For this review, take the finished solid that the model builds, in its own axes (mm). Face numbers are marked on the shaded views. A direction names the side the tool comes from. Round coordinates to 2 decimals unless told otherwise and drop trailing zeros. Write each loop counter-clockwise with the first axis right and the second up, starting at its lowest first coordinate (ties: lowest second). Pieces come first, ordered by that corner, then holes. Notation, with made-up numbers: (61, -24) -> (119, -24) arc R28 ccw to (119, 12) -> close; hole circle Ø10 at (10, 65.25). An arc over 180 degrees is marked (long way). Write item = value, one per line. Start each with the question number.
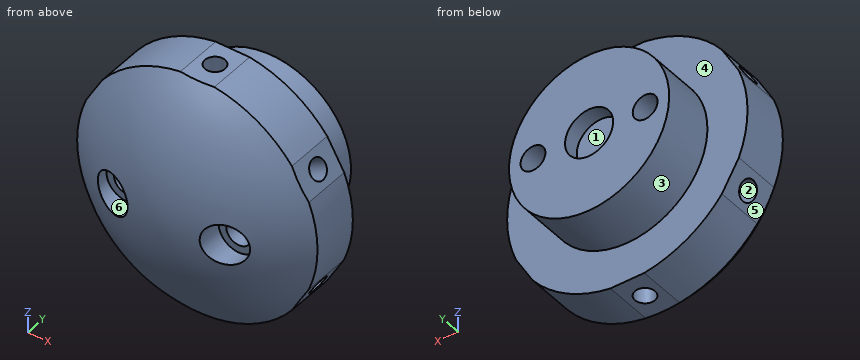
```python
from build123d import *

# Parameters (mm, degrees)
SKETCH_1_R               = 15
EXTRUDE_1_DEPTH          = 6
SKETCH_2_R               = 10
EXTRUDE_2_DEPTH          = 6.5
SKETCH_5_R               = 1.55
CUT_EXTRUDE_967_DEPTH    = 29.287523448
SKETCH_6_R               = 2.5
CUT_EXTRUDE_1129_DEPTH   = 3.7
CUT_EXTRUDE_3_DEPTH      = 25.477792773
PATTERN_CIRCULAR_1_COUNT = 6
SKETCH_12_R              = 3
CUT_EXTRUDE_4_DEPTH      = 2


with BuildPart() as part:
    # 草图1 → 凸台-拉伸1 (new body)
    with BuildSketch(Plane(origin=(0, 0, 0), x_dir=(1, 0, 0), z_dir=(0, 1, 0))):
        with Locations(Location((0, 0, 0), (0, 0, 270))):
            Circle(SKETCH_1_R)
    extrude(amount=EXTRUDE_1_DEPTH)

    # 草图2 → 凸台-拉伸2 (add)
    with BuildSketch(Plane(origin=(0, 6, 0), x_dir=(1, 0, 0), z_dir=(0, 1, 0))):
        with Locations(Location((0, 0, 0), (0, 0, 90))):
            Circle(SKETCH_2_R)
    extrude(amount=EXTRUDE_2_DEPTH)

    # 草图4 → 旋转1 (revolve)
    with BuildSketch(Plane.XY, mode=Mode.PRIVATE) as revolve_1_sk:
        with BuildLine():
            Line((0, 0), (0, -6.213203436))
            ThreePointArc((0, -6.213203436), (8.117941502, -4.598444473), (15, 0))
            Line((15, 0), (0, 0))
        make_face()
    revolve(revolve_1_sk.sketch.rotate(Axis((0, 0, 0), (0, -1, 0)), 180), axis=Axis((0, 0, 0), (0, -1, 0)))

    # 草图5 → Cut-Extrude 967 (cut, through all)
    with BuildSketch(Plane(origin=(0, 12.5, 0), x_dir=(1, 0, 0), z_dir=(0, 1, 0))):
        with Locations(Location((7, 0, 0), (0, 0, 270))):
            Circle(SKETCH_5_R)
        with Locations(Location((-7, 0, 0), (0, 0, 270))):
            Circle(SKETCH_5_R)
    extrude(amount=-CUT_EXTRUDE_967_DEPTH, mode=Mode.SUBTRACT)

    # 草图6 → Cut-Extrude 1129 (cut)
    with BuildSketch(Plane(origin=(0, -6.2, 0), x_dir=(1, 0, 0), z_dir=(0, 1, 0))):
        with Locations(Location((-7, 0, 0), (0, 0, 129.482318069))):
            Circle(SKETCH_6_R)
        with Locations(Location((7, 0, 0), (0, 0, 133.910612472))):
            Circle(SKETCH_6_R)
    extrude(amount=CUT_EXTRUDE_1129_DEPTH, mode=Mode.SUBTRACT)

    # 草图9 → 切除-拉伸3 (cut, through all)
    with BuildSketch(Plane(origin=(0, 6, 0), x_dir=(1, 0, 0), z_dir=(0, 1, 0))):
        with BuildLine():
            Line((11.802472048, 9.257518758), (13.918482445, 5.592481242))
            ThreePointArc((13.918482445, 5.592481242), (12.990381057, 7.5), (11.802472048, 9.257518758))
        make_face()
        with BuildLine():
            Line((-2.116010397, 14.85), (2.116010397, 14.85))
            ThreePointArc((2.116010397, 14.85), (0, 15), (-2.116010397, 14.85))
        make_face()
        with BuildLine():
            Line((13.918482445, -5.592481242), (11.802472048, -9.257518758))
            ThreePointArc((11.802472048, -9.257518758), (12.990381057, -7.5), (13.918482445, -5.592481242))
        make_face()
        with BuildLine():
            Line((2.116010397, -14.85), (-2.116010397, -14.85))
            ThreePointArc((-2.116010397, -14.85), (0, -15), (2.116010397, -14.85))
        make_face()
        with BuildLine():
            Line((-11.802472048, -9.257518758), (-13.918482445, -5.592481242))
            ThreePointArc((-13.918482445, -5.592481242), (-12.990381057, -7.5), (-11.802472048, -9.257518758))
        make_face()
        with BuildLine():
            Line((-13.918482445, 5.592481242), (-11.802472048, 9.257518758))
            ThreePointArc((-11.802472048, 9.257518758), (-12.990381057, 7.5), (-13.918482445, 5.592481242))
        make_face()
    extrude(amount=-CUT_EXTRUDE_3_DEPTH, mode=Mode.SUBTRACT)

    # 草图11 → M3 螺纹孔2 (revolve, cut)
    with BuildSketch(Plane(origin=(-12.860477246, 3, -7.425), x_dir=(-0.50000000000004, 0, 0.8660254037844157), z_dir=(0, 1, 0))):
        Polygon((0, 0), (0, 8.751075774), (1.25, 8), (1.25, 0), align=None)
    hole_wizard_m3_2 = revolve(axis=Axis((-18.35973856, 3, -10.6), (0.8660254037844156, 0, 0.5000000000000397)), mode=Mode.SUBTRACT)

    # 阵列(圆周)1: M3 螺纹孔2 ×6 about axis
    pattern_circular_1_axis = Axis((0, 6, 0), (0, 1, 0))
    for i in range(1, PATTERN_CIRCULAR_1_COUNT):
        add(hole_wizard_m3_2.rotate(pattern_circular_1_axis, i * 360 / PATTERN_CIRCULAR_1_COUNT), mode=Mode.SUBTRACT)

    # 草图12 → 切除-拉伸4 (cut)
    with BuildSketch(Plane(origin=(0, 12.5, 0), x_dir=(1, 0, 0), z_dir=(0, 1, 0))):
        with Locations(Location((0, 0, 0), (0, 0, 270))):
            Circle(SKETCH_12_R)
    extrude(amount=-CUT_EXTRUDE_4_DEPTH, mode=Mode.SUBTRACT)


solid = part.part
```
1. Clearance check with flat-ended pins moving along their axes: pin 1 Ø4 at (y, z) = (2.5, -6) entering from -X; pin 2 Ø6 at (x, z) = (0.5, 6) entering from -Y; pin 3 Ø1.5 at (x, z) = (12, -5.5) entering from +Y. State where each tip first meets the part, or that it passes through.
2. Consider section C-C, the plane x = 6. Give the number of separate pieces and of enclosed holes in the cut face, then the cut area to 3 significant figures.
3. Draft analysis for pull direction Y (two halves, no side actions). For the marked faces 1, 2 and 3, state which applies: +Y half, -Y half, draft (parallel to the pull), parting line (faces both ways), or undercut.
4. Wall thickness on L1, parallel to X at y = 7, z = 0; L2, parallel to Z at x = 10, y = 4; L3, parallel to Y at x = 0, z = -13: over which ranges is each line inside the solid? List them lowest first. Write a range as from..to.
5. Consider section D-D, the plane z = -12.25. Give the boundary of the cut face in (x, y).
6. Consider section B-B, the plane z = 0.5. Give the boundary of the cut face in (x, y), then the cut area to 3 significant figures.
7. Machinability: for the marked faces 4, 5 and 6, which of the approach directions +Z, -Z, +X, -X, +Y, -Y give a long, thin tool a straight path to every point of the face, cutting with its end or side? Answer none if there is none.
8. Consider section A-A, the plane y = 5. Give the boundary of the cut face in (x, z), then the cut area to 3 significant figures.
Outcome:
q1.pin_1 = -14.46
q1.pin_2 = -6
q1.pin_3 = 6
q2.separate_pieces = 2
q2.enclosed_holes = 2
q2.area = 313 mm2
q3.face_1 = +Y half
q3.face_2 = undercut
q3.face_3 = draft
q4.L1 = -10..-8.55, -5.45..5.45, 8.55..10
q4.L2 = -11.18..-6.64, -4.91..4.91, 6.64..11.18
q4.L3 = -1.76..1.75, 4.25..6
q5.outline = (-8.66, 0) arc R17.32 ccw to (8.66, 0) -> (8.66, 6) -> (-8.66, 6) -> close; hole circle Ø2.5 at (0, 3)
q6.outline = (-14.99, 0) arc R21.21 ccw to (-9.45, -3.99) -> (-9.45, -2.5) -> (-8.47, -2.5) -> (-8.47, 12.5) -> (-9.99, 12.5) -> (-9.99, 6) -> (-14.99, 6) -> close; (-5.53, -2.5) -> (-4.55, -2.5) -> (-4.55, -5.71) arc R21.21 ccw to (4.55, -5.71) -> (4.55, -2.5) -> (5.53, -2.5) -> (5.53, 12.5) -> (2.96, 12.5) -> (2.96, 10.5) -> (-2.96, 10.5) -> (-2.96, 12.5) -> (-5.53, 12.5) -> close; (8.47, -2.5) -> (9.45, -2.5) -> (9.45, -3.99) arc R21.21 ccw to (14.99, 0) -> (14.99, 6) -> (9.99, 6) -> (9.99, 12.5) -> (8.47, 12.5) -> close
q6.area = 314 mm2
q7.face_4 = +Y
q7.face_5 = -Z, -X, +Y, -Y
q7.face_6 = -Y
q8.outline = (-13.92, -5.59) -> (-11.8, -9.26) arc R15 ccw to (-2.12, -14.85) -> (2.12, -14.85) arc R15 ccw to (11.8, -9.26) -> (13.92, -5.59) arc R15 ccw to (13.92, 5.59) -> (11.8, 9.26) arc R15 ccw to (2.12, 14.85) -> (-2.12, 14.85) arc R15 ccw to (-11.8, 9.26) -> (-13.92, 5.59) arc R15 ccw to start; hole circle Ø3.1 at (-7, 0); hole circle Ø3.1 at (7, 0)
q8.area = 689 mm2
